Here's how the part is built. I have some questions about the finished solid (model axes, mm). A direction names the side the tool comes from. Round coordinates to 2 decimals unless told otherwise and drop trailing zeros. Write each loop counter-clockwise with the first axis right and the second up, starting at its lowest first coordinate (ties: lowest second). Pieces come first, ordered by that corner, then holes. Notation, with made-up numbers: (5.25, -25) -> (43.25, -25) arc R21 ccw to (43.25, 0) -> close; hole circle Ø3 at (58, 22.25). An arc over 180 degrees is marked (long way). Answer as CSV lines item,"result".
from build123d import *

# Parameters (mm, degrees)
SKETCH1_R           = 14.2875
SKETCH1_R_2         = 0.508
BOSS_EXTRUDE1_DEPTH = 0.8
CUT_EXTRUDE1_START  = -0.8
CUT_EXTRUDE1_DEPTH  = 0.8
CUT_EXTRUDE2_DEPTH  = 21.203596524


with BuildPart() as part:
    # Sketch1 → Boss-Extrude1 (new body)
    with BuildSketch(Plane(origin=(0, 0, 0), x_dir=(1, 0, 0), z_dir=(0, 1, 0))):
        with Locations(Location((0, 0, 0), (0, 0, 270))):
            Circle(SKETCH1_R)
        with Locations(Location((0, 12.192, 0), (0, 0, 270))):
            Circle(SKETCH1_R_2, mode=Mode.SUBTRACT)
        with Locations(Location((8.621045876, 8.621045876, 0), (0, 0, 270))):
            Circle(SKETCH1_R_2, mode=Mode.SUBTRACT)
        with Locations(Location((12.192, 0, 0), (0, 0, 270))):
            Circle(SKETCH1_R_2, mode=Mode.SUBTRACT)
        with Locations(Location((8.621045876, -8.621045876, 0), (0, 0, 270))):
            Circle(SKETCH1_R_2, mode=Mode.SUBTRACT)
        with Locations(Location((0, -12.192, 0), (0, 0, 270))):
            Circle(SKETCH1_R_2, mode=Mode.SUBTRACT)
        with Locations(Location((-8.621045876, -8.621045876, 0), (0, 0, 270))):
            Circle(SKETCH1_R_2, mode=Mode.SUBTRACT)
        with Locations(Location((-12.192, 0, 0), (0, 0, 270))):
            Circle(SKETCH1_R_2, mode=Mode.SUBTRACT)
        with Locations(Location((-8.621045876, 8.621045876, 0), (0, 0, 270))):
            Circle(SKETCH1_R_2, mode=Mode.SUBTRACT)
    extrude(amount=BOSS_EXTRUDE1_DEPTH)

    # Sketch2 → Cut-Extrude1 (cut)
    with BuildSketch(Plane(origin=(0, 0.8, 0), x_dir=(1, 0, 0), z_dir=(0, 1, 0)).offset(CUT_EXTRUDE1_START)):
        with BuildLine():
            ThreePointArc((10.518139842, 9.669611704), (10.102788136, 10.102788136), (9.669611704, 10.518139842))
            Line((9.669611704, 10.518139842), (9.254259999, 10.102788136))
            ThreePointArc((9.254259999, 10.102788136), (9.254259999, 9.254259999), (10.102788136, 9.254259999))
            Line((10.102788136, 9.254259999), (10.518139842, 9.669611704))
        make_face()
        with BuildLine():
            ThreePointArc((14.2875, 0), (14.284348656, 0.300066185), (14.274896015, 0.6))
            Line((14.274896015, 0.6), (13.6875, 0.6))
            ThreePointArc((13.6875, 0.6), (13.0875, 0), (13.6875, -0.6))
            Line((13.6875, -0.6), (14.274896015, -0.6))
            ThreePointArc((14.274896015, -0.6), (14.284348656, -0.300066185), (14.2875, 0))
        make_face()
        with BuildLine():
            ThreePointArc((0.6, 14.274896015), (0, 14.2875), (-0.6, 14.274896015))
            Line((-0.6, 14.274896015), (-0.6, 13.6875))
            ThreePointArc((-0.6, 13.6875), (0, 13.0875), (0.6, 13.6875))
            Line((0.6, 13.6875), (0.6, 14.274896015))
        make_face()
        with BuildLine():
            ThreePointArc((9.669611704, -10.518139842), (10.102788136, -10.102788136), (10.518139842, -9.669611704))
            Line((10.518139842, -9.669611704), (10.102788136, -9.254259999))
            ThreePointArc((10.102788136, -9.254259999), (9.254259999, -9.254259999), (9.254259999, -10.102788136))
            Line((9.254259999, -10.102788136), (9.669611704, -10.518139842))
        make_face()
        with BuildLine():
            Line((-0.6, -13.6875), (-0.6, -14.274896015))
            ThreePointArc((-0.6, -14.274896015), (0, -14.2875), (0.6, -14.274896015))
            Line((0.6, -14.274896015), (0.6, -13.6875))
            ThreePointArc((0.6, -13.6875), (0, -13.0875), (-0.6, -13.6875))
        make_face()
        with BuildLine():
            Line((-10.102788136, -9.254259999), (-10.518139842, -9.669611704))
            ThreePointArc((-10.518139842, -9.669611704), (-10.102788136, -10.102788136), (-9.669611704, -10.518139842))
            Line((-9.669611704, -10.518139842), (-9.254259999, -10.102788136))
            ThreePointArc((-9.254259999, -10.102788136), (-9.254259999, -9.254259999), (-10.102788136, -9.254259999))
        make_face()
        with BuildLine():
            Line((-13.6875, 0.6), (-14.274896015, 0.6))
            ThreePointArc((-14.274896015, 0.6), (-14.2875, 0), (-14.274896015, -0.6))
            Line((-14.274896015, -0.6), (-13.6875, -0.6))
            ThreePointArc((-13.6875, -0.6), (-13.0875, 0), (-13.6875, 0.6))
        make_face()
        with BuildLine():
            Line((-9.254259999, 10.102788136), (-9.669611704, 10.518139842))
            ThreePointArc((-9.669611704, 10.518139842), (-10.102788136, 10.102788136), (-10.518139842, 9.669611704))
            Line((-10.518139842, 9.669611704), (-10.102788136, 9.254259999))
            ThreePointArc((-10.102788136, 9.254259999), (-9.254259999, 9.254259999), (-9.254259999, 10.102788136))
        make_face()
    extrude(amount=CUT_EXTRUDE1_DEPTH, mode=Mode.SUBTRACT)

    # Sketch3 → Cut-Extrude2 (cut, through all)
    with BuildSketch(Plane(origin=(0, 0.8, 0), x_dir=(1, 0, 0), z_dir=(0, 1, 0))):
        with BuildLine():
            Line((-0.508, 2.54), (-0.508, 7.62))
            ThreePointArc((-0.508, 7.62), (0, 8.128), (0.508, 7.62))
            Line((0.508, 7.62), (0.508, 2.54))
            ThreePointArc((0.508, 2.54), (0, 2.032), (-0.508, 2.54))
        make_face()
        with BuildLine():
            Line((0.830059095, 2.453704526), (3.370059095, 6.853113577))
            ThreePointArc((3.370059095, 6.853113577), (4.064, 7.039054482), (4.249940905, 6.345113577))
            Line((4.249940905, 6.345113577), (1.709940905, 1.945704526))
            ThreePointArc((1.709940905, 1.945704526), (1.016, 1.75976362), (0.830059095, 2.453704526))
        make_face()
        with BuildLine():
            Line((1.945704526, 1.709940905), (6.345113577, 4.249940905))
            ThreePointArc((6.345113577, 4.249940905), (7.039054482, 4.064), (6.853113577, 3.370059095))
            Line((6.853113577, 3.370059095), (2.453704526, 0.830059095))
            ThreePointArc((2.453704526, 0.830059095), (1.75976362, 1.016), (1.945704526, 1.709940905))
        make_face()
        with BuildLine():
            Line((2.54, 0.508), (7.62, 0.508))
            ThreePointArc((7.62, 0.508), (8.128, 0), (7.62, -0.508))
            Line((7.62, -0.508), (2.54, -0.508))
            ThreePointArc((2.54, -0.508), (2.032, 0), (2.54, 0.508))
        make_face()
        with BuildLine():
            Line((2.453704526, -0.830059095), (6.853113577, -3.370059095))
            ThreePointArc((6.853113577, -3.370059095), (7.039054482, -4.064), (6.345113577, -4.249940905))
            Line((6.345113577, -4.249940905), (1.945704526, -1.709940905))
            ThreePointArc((1.945704526, -1.709940905), (1.75976362, -1.016), (2.453704526, -0.830059095))
        make_face()
        with BuildLine():
            Line((1.709940905, -1.945704526), (4.249940905, -6.345113577))
            ThreePointArc((4.249940905, -6.345113577), (4.064, -7.039054482), (3.370059095, -6.853113577))
            Line((3.370059095, -6.853113577), (0.830059095, -2.453704526))
            ThreePointArc((0.830059095, -2.453704526), (1.016, -1.75976362), (1.709940905, -1.945704526))
        make_face()
        with BuildLine():
            Line((0.508, -2.54), (0.508, -7.62))
            ThreePointArc((0.508, -7.62), (0, -8.128), (-0.508, -7.62))
            Line((-0.508, -7.62), (-0.508, -2.54))
            ThreePointArc((-0.508, -2.54), (0, -2.032), (0.508, -2.54))
        make_face()
        with BuildLine():
            Line((-0.830059095, -2.453704526), (-3.370059095, -6.853113577))
            ThreePointArc((-3.370059095, -6.853113577), (-4.064, -7.039054482), (-4.249940905, -6.345113577))
            Line((-4.249940905, -6.345113577), (-1.709940905, -1.945704526))
            ThreePointArc((-1.709940905, -1.945704526), (-1.016, -1.75976362), (-0.830059095, -2.453704526))
        make_face()
        with BuildLine():
            Line((-1.945704526, -1.709940905), (-6.345113577, -4.249940905))
            ThreePointArc((-6.345113577, -4.249940905), (-7.039054482, -4.064), (-6.853113577, -3.370059095))
            Line((-6.853113577, -3.370059095), (-2.453704526, -0.830059095))
            ThreePointArc((-2.453704526, -0.830059095), (-1.75976362, -1.016), (-1.945704526, -1.709940905))
        make_face()
        with BuildLine():
            Line((-2.54, -0.508), (-7.62, -0.508))
            ThreePointArc((-7.62, -0.508), (-8.128, 0), (-7.62, 0.508))
            Line((-7.62, 0.508), (-2.54, 0.508))
            ThreePointArc((-2.54, 0.508), (-2.032, 0), (-2.54, -0.508))
        make_face()
        with BuildLine():
            Line((-2.453704526, 0.830059095), (-6.853113577, 3.370059095))
            ThreePointArc((-6.853113577, 3.370059095), (-7.039054482, 4.064), (-6.345113577, 4.249940905))
            Line((-6.345113577, 4.249940905), (-1.945704526, 1.709940905))
            ThreePointArc((-1.945704526, 1.709940905), (-1.75976362, 1.016), (-2.453704526, 0.830059095))
        make_face()
        with BuildLine():
            Line((-1.709940905, 1.945704526), (-4.249940905, 6.345113577))
            ThreePointArc((-4.249940905, 6.345113577), (-4.064, 7.039054482), (-3.370059095, 6.853113577))
            Line((-3.370059095, 6.853113577), (-0.830059095, 2.453704526))
            ThreePointArc((-0.830059095, 2.453704526), (-1.016, 1.75976362), (-1.709940905, 1.945704526))
        make_face()
    extrude(amount=-CUT_EXTRUDE2_DEPTH, mode=Mode.SUBTRACT)


solid = part.part
Item 1: If we mould it in two halves opening along X, with no side actions, what happens to faces 3 (the flat face through (0, 0.8, 0)), 4 (the cylindrical face through (9.26, 0.39, 9.25)), 5 (the cylindrical face through (-13.173, 0.394, -5.532))? For each: pulls with the +X half, pulls with the -X half, needs draft (parallel to the pull), parting line crosses it, or undercut.
Results found:
face 3,"needs draft"
face 4,"undercut"
face 5,"pulls with the -X half"
Item 2: Suppose I cut it at D-D, the plane z = -3.81. List the corners of the cut face in (x, y) for me.
Results found:
outline,"(-13.77, 0) -> (-7.11, 0) -> (-7.11, 0.8) -> (-13.77, 0.8) -> close; (-5.58, 0) -> (-2.79, 0) -> (-2.79, 0.8) -> (-5.58, 0.8) -> close; (-1.61, 0) -> (-0.51, 0) -> (-0.51, 0.8) -> (-1.61, 0.8) -> close; (0.51, 0) -> (1.61, 0) -> (1.61, 0.8) -> (0.51, 0.8) -> close; (2.79, 0) -> (5.58, 0) -> (5.58, 0.8) -> (2.79, 0.8) -> close; (7.11, 0) -> (13.77, 0) -> (13.77, 0.8) -> (7.11, 0.8) -> close"
Item 3: For faces 1 (the flat face through (-3, 0.41, 4.18)), 2 (the cylindrical face through (5.532, 0.394, -13.173)), which set-ups out of +Z, -Z, +X, -X, +Y, -Y let a thin tool reach every point of the face, with its end or its side?
Results found:
face 1,"+Y, -Y"
face 2,"-Z, +X, +Y, -Y"
Item 4: Will this pin go through, and if not, where does the flat tip stop? pin 1 (1.3 mm diameter, centred on x = -12.192, z = 0, fed in from +Y).
Results found:
pin 1,"stops at y = 0.8"
Item 5: Suppose I cut it at C-C, the plane x = 5.75. List the corners of the cut face in (y, z) for me, then the cut area to 3 significant figures.
Results found:
outline,"(0, -13.08) -> (0.8, -13.08) -> (0.8, -3.91) -> (0, -3.91) -> close; (0, -2.73) -> (0.8, -2.73) -> (0.8, -0.51) -> (0, -0.51) -> close; (0, 0.51) -> (0.8, 0.51) -> (0.8, 2.73) -> (0, 2.73) -> close; (0, 3.91) -> (0.8, 3.91) -> (0.8, 13.08) -> (0, 13.08) -> close"
area,"18.2 mm²"
Item 6: Suppose I cut it at B-B, the plane x = -3.81. List the corners of the cut face in (y, z) for me.
Results found:
outline,"(0, -13.77) -> (0.8, -13.77) -> (0.8, -7.11) -> (0, -7.11) -> close; (0, -5.58) -> (0.8, -5.58) -> (0.8, -2.79) -> (0, -2.79) -> close; (0, -1.61) -> (0.8, -1.61) -> (0.8, -0.51) -> (0, -0.51) -> close; (0, 0.51) -> (0.8, 0.51) -> (0.8, 1.61) -> (0, 1.61) -> close; (0, 2.79) -> (0.8, 2.79) -> (0.8, 5.58) -> (0, 5.58) -> close; (0, 7.11) -> (0.8, 7.11) -> (0.8, 13.77) -> (0, 13.77) -> close"
Item 7: Suppose I cut it at A-A, the plane z = 0. List the corners of the cut face in (x, y) for me.
Results found:
outline,"(-13.09, 0) -> (-12.7, 0) -> (-12.7, 0.8) -> (-13.09, 0.8) -> close; (-11.68, 0) -> (-8.13, 0) -> (-8.13, 0.8) -> (-11.68, 0.8) -> close; (-2.03, 0) -> (2.03, 0) -> (2.03, 0.8) -> (-2.03, 0.8) -> close; (8.13, 0) -> (11.68, 0) -> (11.68, 0.8) -> (8.13, 0.8) -> close; (12.7, 0) -> (13.09, 0) -> (13.09, 0.8) -> (12.7, 0.8) -> close"
Item 8: I need wall thicknesses on L1, parallel to X at y = 0.7, z = -4.5; L2, parallel to X at y = 0.3, z = 5; L3, parallel to Z at x = -3.25, y = 0.75. Which ranges of each line are inside material? Lowest first, please.
Results found:
L1,"x = -13.56 to -3.18, -2.01 to -0.51, 0.51 to 2.01, 3.18 to 13.56"
L2,"x = -13.38 to -3.47, -2.3 to -0.51, 0.51 to 2.3, 3.47 to 13.38"
L3,"z = -13.91 to -6.65, -4.61 to -2.46, -1.29 to -0.51, 0.51 to 1.29, 2.46 to 4.61, 6.65 to 13.91"
